Part print with two shaded views. Sizes in mm from the minimum x, y, z corner. Coordinates: 2 decimals unless noted, no trailing zeros. Loops run counter-clockwise (first coordinate to the right, second up) from the corner with the lowest first, then second, coordinate; pieces in that order, holes last.
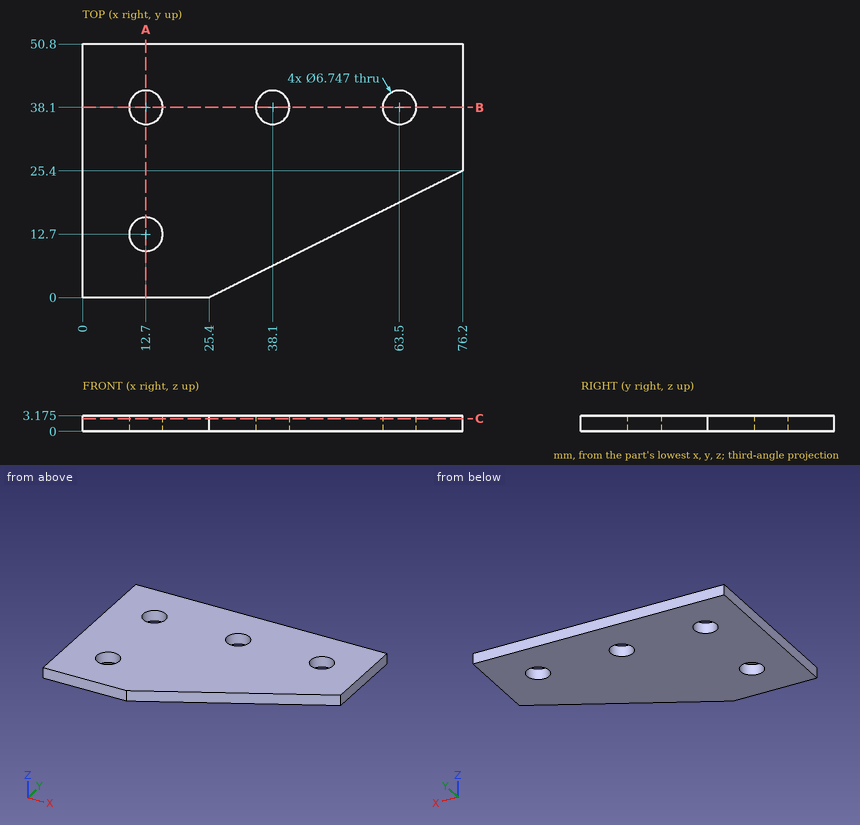
Q1. Slice it at C-C (z = 2.55). List the corners of the cut face in (x, y).
Answers:
outline: (0, 0) - (25.4, 0) - (76.2, 25.4) - (76.2, 50.8) - (0, 50.8) - close; hole circle Ø6.75 at (12.7, 12.7); hole circle Ø6.75 at (12.7, 38.1); hole circle Ø6.75 at (38.1, 38.1); hole circle Ø6.75 at (63.5, 38.1)
Q2. Slice it at B-B (y = 38.1). List the corners of the cut face in (x, z) (1 decimal).
Answers:
outline: (0, 0) - (9.3, 0) - (9.3, 3.2) - (0, 3.2) - close; (16.1, 0) - (34.7, 0) - (34.7, 3.2) - (16.1, 3.2) - close; (41.5, 0) - (60.1, 0) - (60.1, 3.2) - (41.5, 3.2) - close; (66.9, 0) - (76.2, 0) - (76.2, 3.2) - (66.9, 3.2) - close
Q3. Drill centre lines: line 1 (Y direction, x = 11, z = 0.8); line 2 (Y direction, x = 10, z = 2.95); line 3 (X direction, y = 12.5, z = 0.55). Where is each one in solid material? Low to high.
Answers:
line 1: y = 0 to 9.79, 15.61 to 35.19, 41.01 to 50.8
line 2: y = 0 to 10.68, 14.72 to 36.08, 40.12 to 50.8
line 3: x = 0 to 9.33, 16.07 to 50.4
Q4. Slice it at A-A (x = 12.7). List the corners of the cut face in (y, z) (1 decimal), and give its area (3 significant figures).
Answers:
outline: (0, 0) - (9.3, 0) - (9.3, 3.2) - (0, 3.2) - close; (16.1, 0) - (34.7, 0) - (34.7, 3.2) - (16.1, 3.2) - close; (41.5, 0) - (50.8, 0) - (50.8, 3.2) - (41.5, 3.2) - close
area: 118 mm2
Q5. Flat gauge pins, fed straight in: P1, Ø6, axis at x = 12.7, y = 12.7, coming from the -Z side; P2, Ø1.5, axis at x = 51.5, z = 2.5, coming from the -Y side (1 decimal). Where does each tip first touch, or does it go through?
Answers:
P1: passes through
P2: stops at y = 12.7
